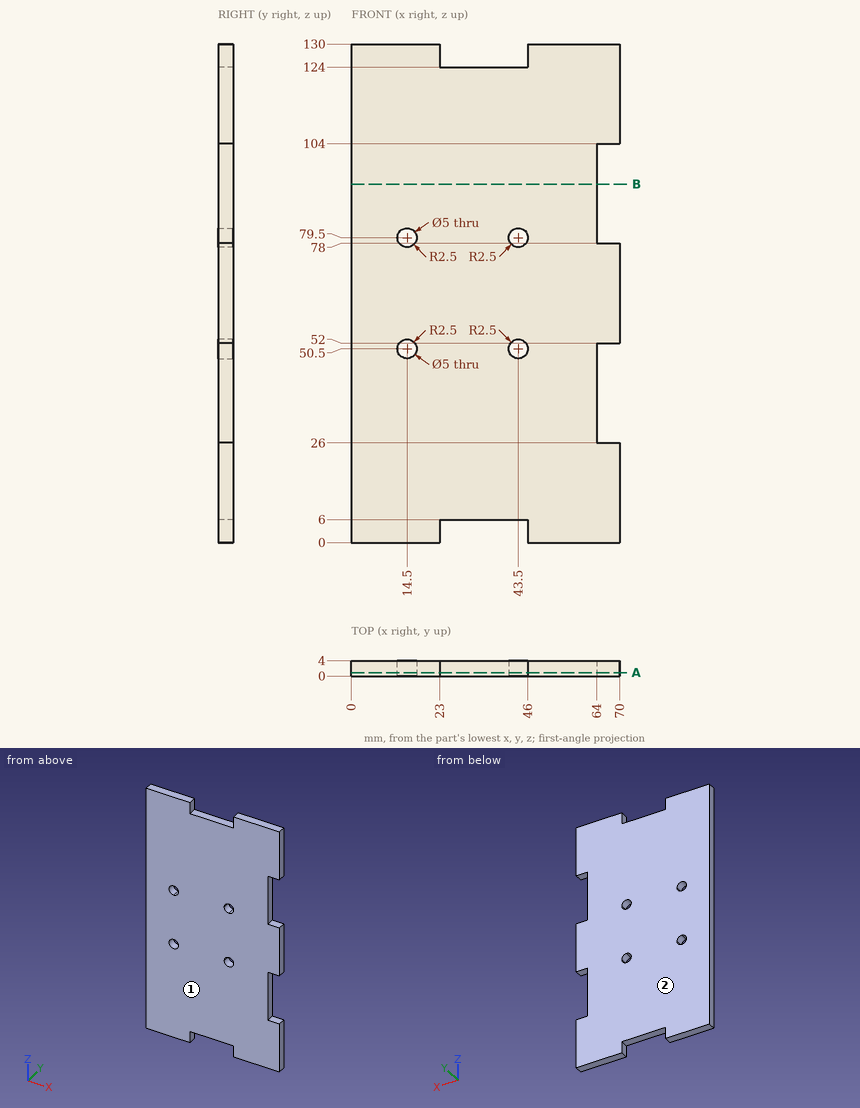
Can you work these out from the drawing? Everything is in mm from the part's minimum corner. Round coordinates to 2 decimals unless told otherwise and drop trailing zeros. Write each loop counter-clockwise with the first axis right and the second up, starting at its lowest first coordinate (ties: lowest second). Pieces come first, ordered by that corner, then holes. Notation, with made-up numbers: M -21.5,-9.75 L -3.5,-9.75 A13 cw -3.5,15.25 Z; hole C -15,-18.75 d2. An arc over 180 degrees is marked long. Use a Markdown table: item, result.
Item 1: I want a section at B-B (z = 93.5). List the corners of the cut face in (x, y) for me, and give its area (3 significant figures).
Found:
| item | result |
|---|---|
| outline | M 0,0 L 64,0 L 64,4 L 0,4 Z |
| area | 256 mm2 |
Item 2: If I drill on line 1 along X through (y, z) = (1.8, 50.5); line 2 along Z through (x, y) = (14.5, 2.25); line 3 along Z through (x, y) = (65, 0.8), over which ranges is the centre line in solid material (lowest first)? Write a range as [from, to].
Found:
| item | result |
|---|---|
| line 1 | x = [0, 12], [17, 41], [46, 64] |
| line 2 | z = [0, 48], [53, 77], [82, 130] |
| line 3 | z = [0, 26], [52, 78], [104, 130] |
Item 3: We'd pull the mould along Y, two halves only. Please class the marked faces 1 and 2: released by +Y, released by -Y, zero draft, split by the parting line, or undercut.
Found:
| item | result |
|---|---|
| face 1 | released by -Y |
| face 2 | released by +Y |
Item 4: For pin 1 Ø1 at (y, z) = (3, 99) entering from +X; pin 2 Ø4 at (x, z) = (14.5, 79.5) entering from +Y, each with a flat end and sliding along its axis, tell me the tip position at first contact or that it passes through.
Found:
| item | result |
|---|---|
| pin 1 | stops at x = 64 |
| pin 2 | passes through |
Item 5: I want a section at A-A (y = 0.9). List the corners of the cut face in (x, z) for me.
Found:
| item | result |
|---|---|
| outline | M 0,0 L 23,0 L 23,6 L 46,6 L 46,0 L 70,0 L 70,26 L 64,26 L 64,52 L 70,52 L 70,78 L 64,78 L 64,104 L 70,104 L 70,130 L 46,130 L 46,124 L 23,124 L 23,130 L 0,130 Z; hole C 14.5,50.5 d5; hole C 14.5,79.5 d5; hole C 43.5,50.5 d5; hole C 43.5,79.5 d5 |
